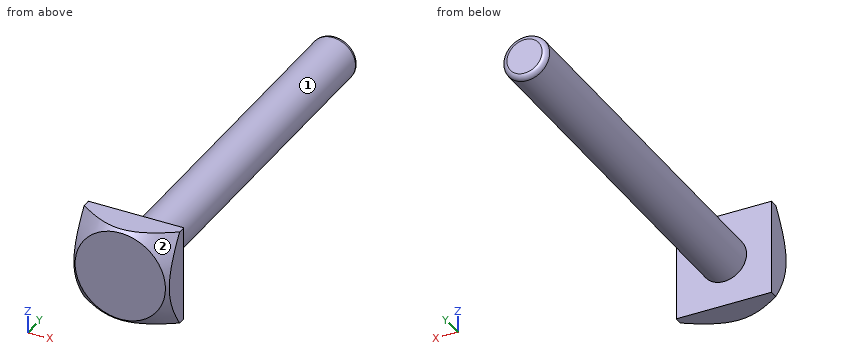
```python
from build123d import *

# Parameters (mm, degrees)
SKETCH1_W           = 19
SKETCH1_H           = 19
BOSS_EXTRUDE1_DEPTH = 6
SKETCH2_R           = 4.5
BOSS_EXTRUDE2_DEPTH = 76
SKETCH3_OUTSIDE_W   = 190.258
SKETCH3_OUTSIDE_H   = 190.258
SKETCH3_OUTSIDE_R   = 9
CUT_EXTRUDE1_DEPTH  = 76
CUT_EXTRUDE1_DRAFT  = -45
FILLET1_R           = 1


with BuildPart() as part:
    # Sketch1 → Boss-Extrude1 (new body)
    with BuildSketch(Plane(origin=(0, 0, 0), x_dir=(1, 0, 0), z_dir=(0, 1, 0))):
        Rectangle(SKETCH1_W, SKETCH1_H)
    extrude(amount=BOSS_EXTRUDE1_DEPTH)

    # Sketch2 → Boss-Extrude2 (add)
    with BuildSketch(Plane(origin=(0, 6, 0), x_dir=(1, 0, 0), z_dir=(0, 1, 0))):
        with Locations(Location((0, 0, 0), (0, 0, 90))):  # turned: the seam where the file's is
            Circle(SKETCH2_R)
    extrude(amount=BOSS_EXTRUDE2_DEPTH)


with BuildPart() as cut_extrude1_tool:
    # Sketch3 outside → Cut-Extrude1 (with draft: the straight prism first)
    with BuildSketch(Plane.XZ):
        Rectangle(SKETCH3_OUTSIDE_W, SKETCH3_OUTSIDE_H)
        Circle(SKETCH3_OUTSIDE_R, mode=Mode.SUBTRACT)
    extrude(amount=-CUT_EXTRUDE1_DEPTH)
    # Cut-Extrude1: the draft: its side faces are tilted about the plane it starts from
    cut_extrude1_sides = [cut_extrude1_tool.faces().sort_by_distance(p)[0] for p in [
        (0, 38, -95.129),
        (95.129, 38, 0),
        (0, 38, 95.129),
        (-95.129, 38, 0),
        (-9, 38, 0),
    ]]
    draft(cut_extrude1_sides, Plane.XZ, CUT_EXTRUDE1_DRAFT)


with BuildPart() as part_1:
    add(part.part)

    # Cut-Extrude1: cut by cut_extrude1_tool
    add(cut_extrude1_tool.part, mode=Mode.SUBTRACT)

    # Fillet1
    fillet1_edges = [part_1.edges().sort_by_distance(p)[0] for p in [
        (0, 82, 4.5),
    ]]
    fillet(fillet1_edges, radius=FILLET1_R)


solid = part_1.part
```
Input: part model. Units: mm. Frame: model coordinates. Face numbers are marked on the shaded views. A direction names the side the tool comes from. Give positions to 0.01 mm unless a question says otherwise; leave off trailing zeros. Write each loop counter-clockwise with the first axis right and the second up, starting at its lowest first coordinate (ties: lowest second). Pieces come first, ordered by that corner, then holes. Notation, with made-up numbers: (24.5, 32.5) - (58.5, 32.5) arc R6 cw to (58.5, 38.5) - close; hole circle Ø10 at (88.25, -20). An arc over 180 degrees is marked (long way). Write item = value, one per line. Start each with the question number.
1. Section query A-A, the plane z = 0. Output: boundary loops of the cut face in (x, y), then the cut area to 3 significant figures.
2. First-contact query: pin 1 Ø8 at (y, z) = (54, 6.5) entering from -X; pin 2 Ø5 at (x, y) = (0.5, 70) entering from -Z; pin 3 Ø4 at (x, y) = (5, 72) entering from +Z. Flat tips, straight axial feed; report the tip coordinate or a pass-through.
3. Ray query, L1, parallel to Y at x = -7, z = 4.25; L2, parallel to Y at x = -3.25, z = -1.5; L3, parallel to Z at x = 0.25, y = 57.5. Return the intervals inside material, ascending.
4. Access query for the marked faces 1 and 2. Directions: +Z, -Z, +X, -X, +Y, -Y. A direction counts if a zero-diameter tool reaches every point of the face in a straight line with its end or side. Return the directions, or none.
5. Section query C-C, the plane y = 64. Output: boundary loops of the cut face in (x, z).
6. Section query B-B, the plane x = 0. Output: boundary loops of the cut face in (y, z).
Check sheet entries:
q1.outline = (-9.5, 0.5) - (-9, 0) - (9, 0) - (9.5, 0.5) - (9.5, 6) - (4.5, 6) - (4.5, 81) arc R1 ccw to (3.5, 82) - (-3.5, 82) arc R1 ccw to (-4.5, 81) - (-4.5, 6) - (-9.5, 6) - close
q1.area = 797 mm2
q2.pin_1 = -3.74
q2.pin_2 = -4.5
q2.pin_3 = 3.35
q3.L1 = 0 to 6
q3.L2 = 0 to 82
q3.L3 = -4.49 to 4.49
q4.face_1 = +Y
q4.face_2 = -Y
q5.outline = circle Ø9 at (0, 0)
q6.outline = (0, -9) - (0.5, -9.5) - (6, -9.5) - (6, -4.5) - (81, -4.5) arc R1 ccw to (82, -3.5) - (82, 3.5) arc R1 ccw to (81, 4.5) - (6, 4.5) - (6, 9.5) - (0.5, 9.5) - (0, 9) - close
